Check sheet for the drawn part. Datum: minimum x, y, z corner. Units: mm. A direction names the side the tool comes from. Coordinates: 2 decimals unless noted, no trailing zeros. Write each loop counter-clockwise with the first axis right and the second up, starting at its lowest first coordinate (ties: lowest second). Pieces come first, ordered by that corner, then holes. Notation, with made-up numbers: (-34.5, -13) - (8.5, -13) arc R14 ccw to (8.5, 6) - close; hole circle Ø9 at (70, 18). An arc over 180 degrees is marked (long way). Use one line per item in the form item = value. Start each with the question number.
1. Cross-section at A-A on x = 10.5. Record the boundary of the cut face in (y, z).
2. Cross-section at B-B on z = 10.5. Record the boundary of the cut face in (x, y).
3. Scan lines: line 1 along X through (y, z) = (9, 10.5); line 2 along X through (y, z) = (1.75, 17.5); line 3 along Y through (x, z) = (15, 2). Record each from-to range of solid material in increasing order.
4. Cross-section at C-C on z = 13.75. Record the boundary of the cut face in (x, y), then the cut area to 3 significant figures.
5. Cross-section at D-D on x = 7.25. Record the boundary of the cut face in (y, z), then the cut area to 3 significant figures.
6. Go/stop test with flat-tipped pins: pin 1 Ø8 at (x, z) = (10, 16.5) entering from -Y; pin 2 Ø4 at (x, y) = (14, 12.5) entering from +Z; pin 3 Ø2 at (y, z) = (14.5, 14) entering from -X; pin 4 Ø1.5 at (y, z) = (19, 8.5) entering from -X. Record where each tip stops, or that it passes through.
7. Tool access check on the marked faces 1 and 2. Record the directions out of +Z, -Z, +X, -X, +Y, -Y that give a thin tool (end or side, any length) a straight path to the whole face; none if there is none.
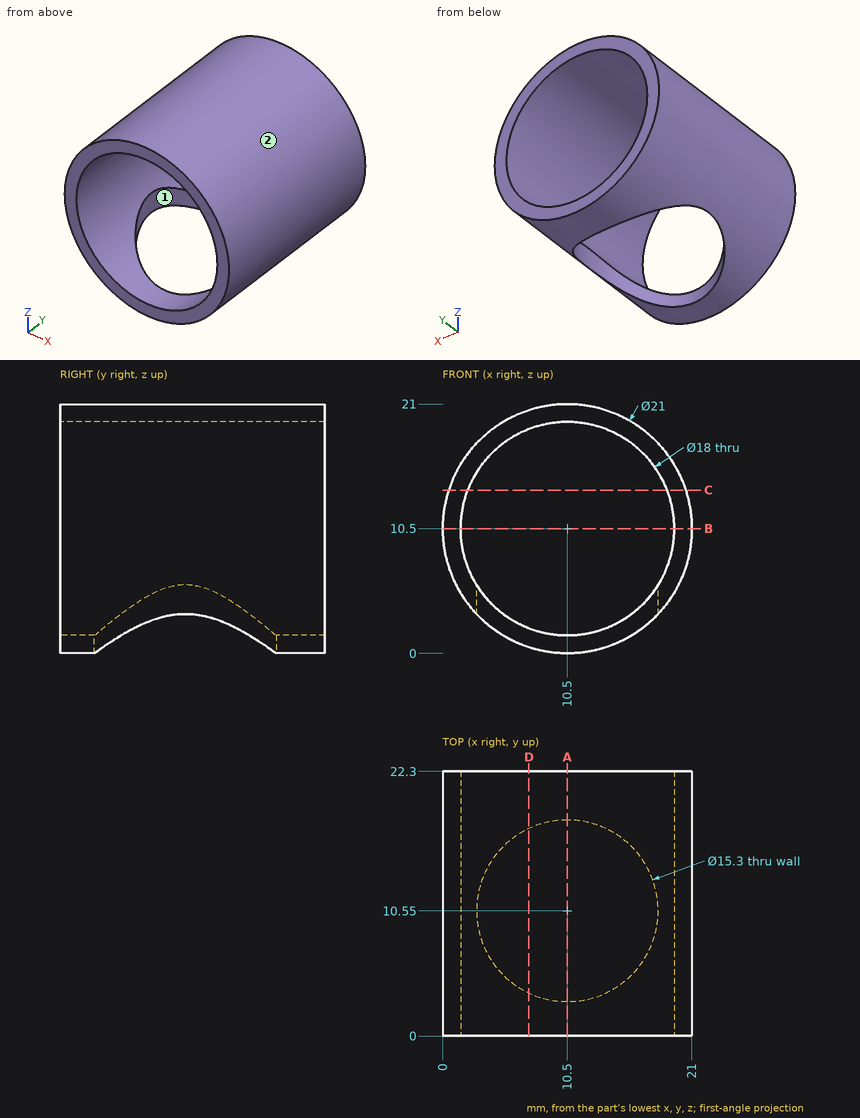
Final values:
q1.outline = (0, 0) - (2.9, 0) - (2.9, 1.5) - (0, 1.5) - close; (0, 19.5) - (22.3, 19.5) - (22.3, 21) - (0, 21) - close; (18.2, 0) - (22.3, 0) - (22.3, 1.5) - (18.2, 1.5) - close
q2.outline = (0, 0) - (1.5, 0) - (1.5, 22.3) - (0, 22.3) - close; (19.5, 0) - (21, 0) - (21, 22.3) - (19.5, 22.3) - close
q3.line_1 = 0 to 1.5, 19.5 to 21
q3.line_2 = 2.67 to 4.84, 16.16 to 18.33
q3.line_3 = 0 to 4.36, 16.74 to 22.3
q4.outline = (0.52, 0) - (2.11, 0) - (2.11, 22.3) - (0.52, 22.3) - close; (18.89, 0) - (20.48, 0) - (20.48, 22.3) - (18.89, 22.3) - close
q4.area = 71.0 mm²
q5.outline = (0, 0.52) - (3.62, 0.52) - (3.62, 2.11) - (0, 2.11) - close; (0, 18.89) - (22.3, 18.89) - (22.3, 20.48) - (0, 20.48) - close; (17.48, 0.52) - (22.3, 0.52) - (22.3, 2.11) - (17.48, 2.11) - close
q5.area = 48.9 mm²
q6.pin_1 = 0
q6.pin_2 = 20.89
q6.pin_3 = 0.3
q6.pin_4 = 0.07
q7.face_1 = -Z
q7.face_2 = +Y, -Y
